The listing builds one solid part. Answer for the finished solid, in the listing's coordinates (mm). Face numbers are marked on the shaded views. A direction names the side the tool comes from. Coordinates: 2 decimals unless noted, no trailing zeros. Order: outer loops, then holes, each group sorted by start corner. A loop starts at its lowest first (then second) coordinate and runs counter-clockwise, first axis right, second up. Notation, with made-up numbers: (-7, 17) -> (23, 17) arc R15 ccw to (23, 26) -> close; hole circle Ø5 at (-29.5, 34). An arc over 180 degrees is marked (long way). Write item = value, one per line.
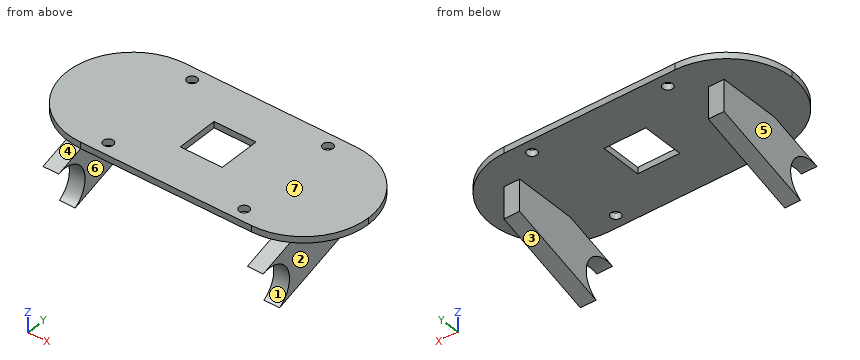
from build123d import *

# Parameters (mm, degrees)
SKETCH1_W           = 191.262
SKETCH1_H           = 82.55
SKETCH1_R           = 3.175
SKETCH1_W_2         = 26.67
SKETCH1_H_2         = 26.67
BOSS_EXTRUDE1_DEPTH = 4
FILLET5_R           = 41.275
BOSS_EXTRUDE2_DEPTH = 10
LPATTERN1_COUNT     = 2
LPATTERN1_PITCH     = 130


with BuildPart() as part:
    # Sketch1 → Boss-Extrude1 (new body)
    with BuildSketch(Plane.XY):
        Rectangle(SKETCH1_W, SKETCH1_H)
        with Locations((-43.18, 33.02)):
            Circle(SKETCH1_R, mode=Mode.SUBTRACT)
        with Locations((43.18, 33.02)):
            Circle(SKETCH1_R, mode=Mode.SUBTRACT)
        with Locations((43.18, -33.02)):
            Circle(SKETCH1_R, mode=Mode.SUBTRACT)
        with Locations((-43.18, -33.02)):
            Circle(SKETCH1_R, mode=Mode.SUBTRACT)
        Rectangle(SKETCH1_W_2, SKETCH1_H_2, mode=Mode.SUBTRACT)
    extrude(amount=BOSS_EXTRUDE1_DEPTH)

    # Fillet5
    fillet5_edges = [part.edges().sort_by_distance(p)[0] for p in [
        (-95.631, -41.275, 2),
        (95.631, -41.275, 2),
        (95.631, 41.275, 2),
        (-95.631, 41.275, 2),
    ]]
    fillet(fillet5_edges, radius=FILLET5_R - 0.0001)  # a hair under: the kernel refuses the full size

    # Sketch2 → Boss-Extrude2 (add)
    with BuildSketch(Plane(origin=(71.59, 0, 0), x_dir=(0, 0, -1), z_dir=(1, 0, 0))):
        with BuildLine():
            Line((0, 20), (20, 20))
            Line((20, 20), (39.561185263, -40.310839577))
            ThreePointArc((39.561185263, -40.310839577), (19.368102567, -33.925421898), (10.798120439, -53.292650765))
            Line((10.798120439, -53.292650765), (0, -20))
            Line((0, -20), (0, 20))
        make_face()
    boss_extrude2 = extrude(amount=-BOSS_EXTRUDE2_DEPTH)

    # LPattern1: Boss-Extrude2 ×2
    with Locations(*[(-i * LPATTERN1_PITCH, 0, 0) for i in range(1, LPATTERN1_COUNT)]):
        add(boss_extrude2)


solid = part.part
Q1. Each of these flat-tipped pins is pushed along its axis until it touches: pin 1 Ø2 at (y, z) = (-14, -22) entering from -X; pin 2 Ø6 at (x, y) = (58, -10.5) entering from -Z; pin 3 Ø12 at (y, z) = (-13.5, -15.5) entering from +X; pin 4 Ø1.5 at (x, z) = (-7.5, -2) entering from +Y. Where does it stop, or does it pass through?
The answers:
pin_1 = -68.41
pin_2 = 0
pin_3 = 71.59
pin_4 = through
Q2. Section C-C, the plane z = -35.5 is taken. Give the vertices of the cut face in (x, y), plus the area to 3 significant figures.
The answers:
outline = (-68.41, -35.75) -> (-58.41, -35.75) -> (-58.41, -27.79) -> (-68.41, -27.79) -> close; (61.59, -35.75) -> (71.59, -35.75) -> (71.59, -27.79) -> (61.59, -27.79) -> close
area = 159 mm2
Q3. Section A-A, the plane x = -9 is taken. Give the vertices of the cut face in (y, z) (3 decimals), plus the area to 3 significant figures.
The answers:
outline = (-41.275, 0) -> (-13.335, 0) -> (-13.335, 4) -> (-41.275, 4) -> close; (13.335, 0) -> (41.275, 0) -> (41.275, 4) -> (13.335, 4) -> close
area = 224 mm2
Q4. Section B-B, the plane x = 43.18 is taken. Give the vertices of the cut face in (y, z) (3 decimals).
The answers:
outline = (-41.275, 0) -> (-36.195, 0) -> (-36.195, 4) -> (-41.275, 4) -> close; (-29.845, 0) -> (29.845, 0) -> (29.845, 4) -> (-29.845, 4) -> close; (36.195, 0) -> (41.275, 0) -> (41.275, 4) -> (36.195, 4) -> close
Q5. Section D-D, the plane y = 33.02 is taken. Give the vertices of the cut face in (x, z) (3 decimals), plus the area to 3 significant figures.
The answers:
outline = (-79.121, 0) -> (-46.355, 0) -> (-46.355, 4) -> (-79.121, 4) -> close; (-40.005, 0) -> (40.005, 0) -> (40.005, 4) -> (-40.005, 4) -> close; (46.355, 0) -> (79.121, 0) -> (79.121, 4) -> (46.355, 4) -> close
area = 582 mm2
Q6. Find the intervals of material crossed by line 1 along Y through (x, z) = (-43.18, 1.55) (3 decimals); line 2 along X through (y, z) = (-9, -19.5); line 3 along X through (y, z) = (33, 2), in increasing order.
The answers:
line_1 = -41.275 to -36.195, -29.845 to 29.845, 36.195 to 41.275
line_2 = -68.41 to -58.41, 61.59 to 71.59
line_3 = -79.15 to -46.35, -40.01 to 40.01, 46.35 to 79.15
Q7. A tool of negligible diameter and unlimited length cuts with its end or side. For the marked faces 5, 6 and 7, from which of +Z, -Z, +X, -X, +Y, -Y can it reach the whole face along a straight path? Write none if from no direction.
The answers:
face_5 = -Z, -X, +Y, -Y
face_6 = -Z, +Y, -Y
face_7 = +Z, +X, -X, +Y, -Y
Q8. The mould has two halves that part along Z. Classify the marked faces 1, 2, 3 and 4: released by +Z, released by -Z, zero draft, split by the parting line, or undercut.
The answers:
face_1 = undercut
face_2 = zero draft
face_3 = released by -Z
face_4 = undercut
